```python
from build123d import *

# Parameters (mm, degrees)
EXTRUDE_1_DEPTH     = 8
SKETCH_2_R          = 1.65
CUT_EXTRUDE_1_DEPTH = 8
SKETCH_3_R          = 2.85
CUT_EXTRUDE_2_DEPTH = 8


with BuildPart() as part:
    # 草图1 → 凸台-拉伸1 (new body)
    with BuildSketch(Plane.XY):
        Polygon((0, 0), (0, -15), (-5, -15), (-5, 5), (20, 5), (20, 0), align=None)
    extrude(amount=EXTRUDE_1_DEPTH)

    # 草图2 → 切除-拉伸1 (cut)
    with BuildSketch(Plane.XZ):
        with Locations((15.65, 4)):
            Circle(SKETCH_2_R)
    extrude(amount=-CUT_EXTRUDE_1_DEPTH, mode=Mode.SUBTRACT)

    # 草图3 → 切除-拉伸2 (cut)
    with BuildSketch(Plane.ZY.offset(5)):
        with Locations(Location((4, -7, 0), (0, 0, 270))):
            Circle(SKETCH_3_R)
    extrude(amount=-CUT_EXTRUDE_2_DEPTH, mode=Mode.SUBTRACT)


solid = part.part
```
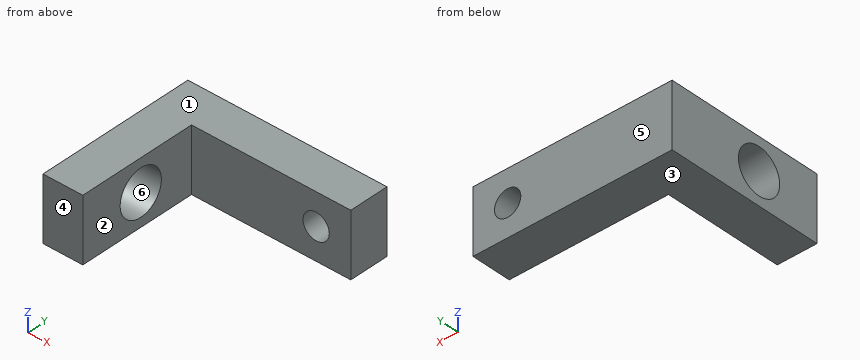
The model under review builds one solid part; all positions refer to its coordinate system, in mm. Face numbers are marked on the shaded views. A direction names the side the tool comes from. Round coordinates to 2 decimals unless told otherwise and drop trailing zeros. Order: outer loops, then holes, each group sorted by start corner. A loop starts at its lowest first (then second) coordinate and runs counter-clockwise, first axis right, second up.
Item 1: Add section A-A, the plane x = 15.65. State the section outline as (y, z) points, and give its area (3 significant figures).
Working result:
outline: (0, 0) - (5, 0) - (5, 2.35) - (0, 2.35) - close; (0, 5.65) - (5, 5.65) - (5, 8) - (0, 8) - close
area: 23.5 mm2
Item 2: Machinability: for the marked faces 1 and 2, which of the approach directions +Z, -Z, +X, -X, +Y, -Y give a long, thin tool a straight path to every point of the face, cutting with its end or side? Answer none if there is none.
Working result:
face 1: +Z, +X, -X, +Y, -Y
face 2: +Z, -Z, +X, -Y
Item 3: To check wall thickness, follow probe 1 along Z at (x, y) = (15.65, 2.6); probe 2 along Z at (x, y) = (-3.6, -7); probe 3 along Y at (x, z) = (0.5, 7.5). State the ranges of each line that lie inside material, in increasing order.
Working result:
probe 1: z = 0 to 2.35, 5.65 to 8
probe 2: z = 0 to 1.15, 6.85 to 8
probe 3: y = 0 to 5
Item 4: For pin 1 (4.5 mm diameter, centred on x = 15.65, z = 4, fed in from -Y), flat-tipped, find the tip position at first contact; note if it passes through.
Working result:
pin 1: stops at y = 0
Item 5: Add section C-C, the plane x = -3.25. State the section outline as (y, z) points, and give its area (3 significant figures).
Working result:
outline: (-15, 0) - (5, 0) - (5, 8) - (-15, 8) - close; hole circle Ø5.7 at (-7, 4)
area: 134 mm2
Item 6: Add section D-D, the plane z = 4.5. State the section outline as (x, y) points, and give its area (3 significant figures).
Working result:
outline: (-5, -15) - (0, -15) - (0, -9.81) - (-5, -9.81) - close; (-5, -4.19) - (0, -4.19) - (0, 0) - (14.08, 0) - (14.08, 5) - (-5, 5) - close; (17.22, 0) - (20, 0) - (20, 5) - (17.22, 5) - close
area: 156 mm2
Item 7: Draft analysis for pull direction Y (two halves, no side actions). For the marked faces 3, 4, 5 and 6, state which applies: released by +Y, released by -Y, zero draft, split by the parting line, or undercut.
Working result:
face 3: zero draft
face 4: released by -Y
face 5: released by +Y
face 6: undercut
Item 8: Add section B-B, the plane y = -7. State the section outline as (x, z) points.
Working result:
outline: (-5, 0) - (0, 0) - (0, 1.15) - (-5, 1.15) - close; (-5, 6.85) - (0, 6.85) - (0, 8) - (-5, 8) - close
